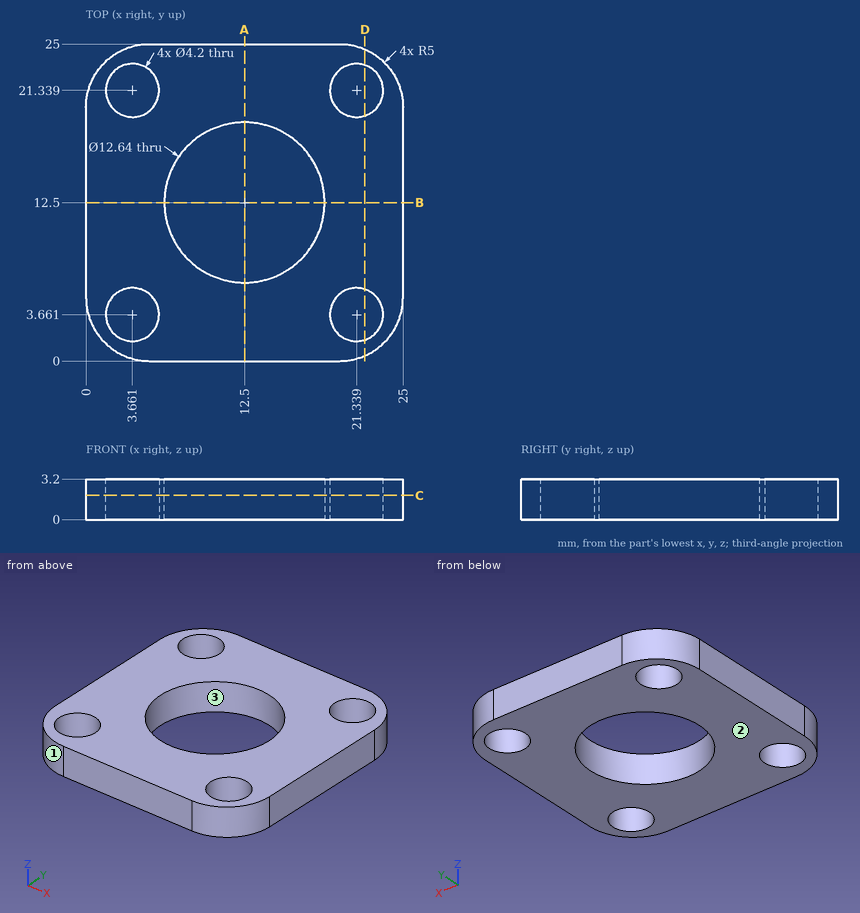
Study the drawing (mm; zero at the part's minimum x, y, z) and answer. Round coordinates to 2 decimals unless told otherwise and drop trailing zeros. Write each loop counter-clockwise with the first axis right and the second up, starting at its lowest first coordinate (ties: lowest second). Pieces come first, ordered by that corner, then holes.
1) A cutting plane is placed at D-D on x = 22. Determine the outline of the cut face in (y, z).
2) A cutting plane is placed at C-C on z = 1.9. Determine the outline of the cut face in (x, y), and give its area (3 significant figures).
3) A cutting plane is placed at A-A on x = 12.5. Determine the outline of the cut face in (y, z).
4) Consider probe 1 along Y at (x, z) = (22.25, 1.55) (1 decimal); probe 2 along X at (y, z) = (19.75, 0.9) (1 decimal); probe 3 along Y at (x, z) = (5.5, 0.5) (1 decimal). Determine where each line is inside the solid, lowest interval first.
5) Determine the mould class of the marked faces 1, 2 and 3 for opening direction Y: pulls with the +Y half, pulls with the -Y half, needs draft (parallel to the pull), parting line crosses it, or undercut.
Entries:
1. outline: (0.42, 0) - (1.67, 0) - (1.67, 3.2) - (0.42, 3.2) - close; (5.65, 0) - (19.35, 0) - (19.35, 3.2) - (5.65, 3.2) - close; (23.33, 0) - (24.58, 0) - (24.58, 3.2) - (23.33, 3.2) - close
2. outline: (0, 5) arc R5 ccw to (5, 0) - (20, 0) arc R5 ccw to (25, 5) - (25, 20) arc R5 ccw to (20, 25) - (5, 25) arc R5 ccw to (0, 20) - close; hole circle Ø4.2 at (3.66, 3.66); hole circle Ø4.2 at (3.66, 21.34); hole circle Ø12.64 at (12.5, 12.5); hole circle Ø4.2 at (21.34, 3.66); hole circle Ø4.2 at (21.34, 21.34)
2. area: 423 mm2
3. outline: (0, 0) - (6.18, 0) - (6.18, 3.2) - (0, 3.2) - close; (18.82, 0) - (25, 0) - (25, 3.2) - (18.82, 3.2) - close
4. probe 1: y = 0.5 to 1.8, 5.6 to 19.4, 23.2 to 24.5
4. probe 2: x = 0 to 2.3, 5 to 20, 22.7 to 25
4. probe 3: y = 0 to 2.6, 4.7 to 20.3, 22.4 to 25
5. face 1: pulls with the -Y half
5. face 2: needs draft
5. face 3: undercut
